Can you work these out from the model? Positions are in its coordinate system, mm. Face numbers are marked on the shaded views. A direction names the side the tool comes from. Give positions to 0.01 mm unless a question says otherwise; leave off trailing zeros. Write each loop counter-clockwise with the first axis right and the second up, starting at its lowest first coordinate (ties: lowest second). Pieces come first, ordered by that corner, then holes.
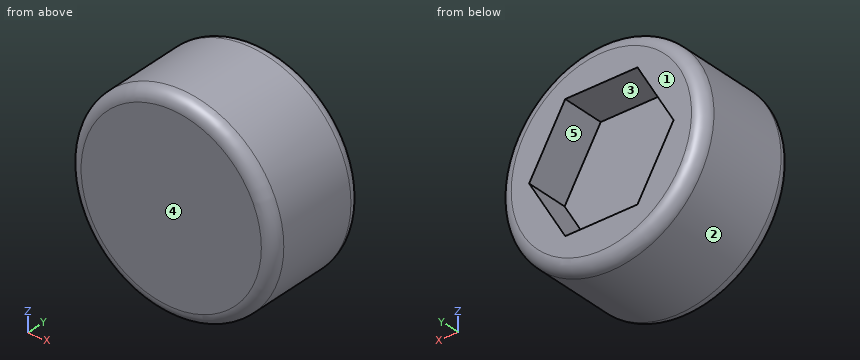
from build123d import *

# Parameters (mm, degrees)
F0_R     = 84.46775
F1_DEPTH = 87.570764
F2_R     = 10.16
F4_DEPTH = 35.56


with BuildPart() as f1:
    # F0 (on Front) → F1 (new body)
    with BuildSketch(Plane.XZ):
        Circle(F0_R)
    extrude(amount=F1_DEPTH)

    # F2
    f2_edges = [f1.edges().sort_by_distance(p)[0] for p in [
        (-84.46775, -87.570764, 0),
        (-84.46775, 0, 0),
    ]]
    fillet(f2_edges, radius=F2_R)

    # F3 (on face) → F4 (cut)
    with BuildSketch(Plane(origin=(0, 0, 0), x_dir=(-1, 0, 0), z_dir=(0, 1, 0))):
        Polygon((29.785042, 51.589206), (-29.785042, 51.589206), (-59.570084, 0), (-29.785042, -51.589206), (29.785042, -51.589206), (59.570084, 0), align=None)
    extrude(amount=-F4_DEPTH, mode=Mode.SUBTRACT)


solid = f1.part
(1) For the marked faces 4 and 5, which set-ups out of +Z, -Z, +X, -X, +Y, -Y let a thin tool reach every point of the face, with its end or its side?
Returned:
face 4: +Z, -Z, +X, -X, -Y
face 5: +Y
(2) Imagine slicing it at C-C, the plane y = -80.5. Write out the boundary of the cut face in (x, z).
Returned:
outline: circle Ø167.97 at (0, 0)
(3) If I drill on L1, parallel to Y at x = -29, z = -39; L2, parallel to Z at x = -35.5, y = -15; L3, parallel to Z at x = -24.5, y = -11, over which ranges is the centre line in solid material (lowest first)?
Returned:
L1: y = -87.57 to -35.56
L2: z = -76.65 to -41.69, 41.69 to 76.65
L3: z = -80.84 to -51.59, 51.59 to 80.84
(4) Will these pins go through, and if not, where does the flat tip stop? P1, Ø3, axis at x = 10.5, y = -69, coming from the +Z side; P2, Ø5, axis at x = -13, y = -35.5, coming from the +Z side; P3, Ø4, axis at y = -32, z = -55.5, coming from the +X side.
Returned:
P1: stops at z = 83.99
P2: stops at z = 83.81
P3: stops at x = 65.36
(5) If we mould it in two halves opening along Z, with no side actions, what happens to the marked faces 1, 2 and 3? For each: +Z half, -Z half, draft (parallel to the pull), parting line (faces both ways), or undercut.
Returned:
face 1: draft
face 2: parting line
face 3: undercut
(6) Imagine slicing it at B-B, the plane y = -67. Write out the boundary of the cut face in (x, z), plus the area to 3 significant figures.
Returned:
outline: circle Ø168.94 at (0, 0)
area: 22,400 mm2
(7) Imagine slicing it at A-A, the plane x = 0. Write out the boundary of the cut face in (y, z), plus the area to 3 significant figures.
Returned:
outline: (-87.57, -74.31) arc R10.16 ccw to (-77.41, -84.47) - (-10.16, -84.47) arc R10.16 ccw to (0, -74.31) - (0, -51.59) - (-35.56, -51.59) - (-35.56, 51.59) - (0, 51.59) - (0, 74.31) arc R10.16 ccw to (-10.16, 84.47) - (-77.41, 84.47) arc R10.16 ccw to (-87.57, 74.31) - close
area: 11,000 mm2
